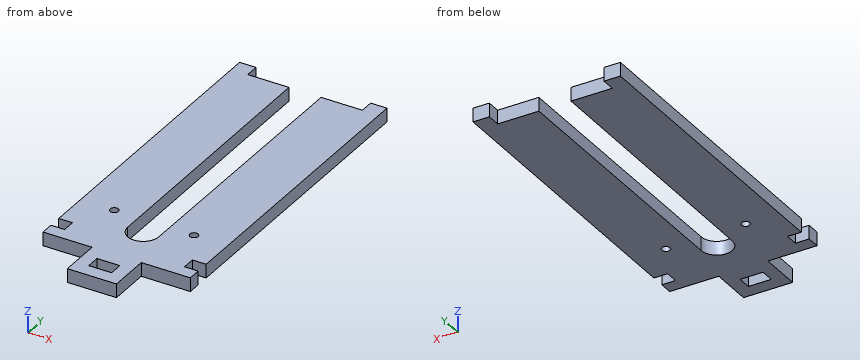
```python
from build123d import *

# Parameters (mm, degrees)
SKETCH1_W           = 57.15
SKETCH1_H           = 127
BOSS_EXTRUDE3_DEPTH = 5.334
CUT_EXTRUDE2_DEPTH  = 140.368483008
SKETCH8_W           = 19.05
SKETCH8_H           = 5.334
CUT_EXTRUDE6_DEPTH  = 5.334
SKETCH8_5_W         = 19.05
SKETCH8_5_H         = 5.334
CUT_EXTRUDE7_DEPTH  = 5.334
SKETCH16_W          = 22.352
SKETCH16_H          = 5.334
BOSS_EXTRUDE4_DEPTH = 5.334
SKETCH32_W          = 16.002
SKETCH32_H          = 5.334
CUT_EXTRUDE13_DEPTH = 5.334
SKETCH35_R          = 1.6
CUT_EXTRUDE15_DEPTH = 145.245837417
SKETCH36_W          = 19.05
SKETCH36_H          = 5.334
BOSS_EXTRUDE5_DEPTH = 10.668
SKETCH37_W          = 8.89
SKETCH37_H          = 5.334
CUT_EXTRUDE16_DEPTH = 145.245837417
SKETCH38_W          = 5.334
SKETCH38_H          = 5.08
CUT_EXTRUDE17_DEPTH = 145.245837417


with BuildPart() as part:
    # Sketch1 → Boss-Extrude3 (new body)
    with BuildSketch(Plane.XY):
        with Locations((28.575, 63.5)):
            Rectangle(SKETCH1_W, SKETCH1_H)
    extrude(amount=BOSS_EXTRUDE3_DEPTH)

    # Sketch3 → Cut-Extrude2 (cut, through all)
    with BuildSketch(Plane.XY.offset(5.334)):
        with BuildLine():
            Line((34.798, 127), (22.352, 127))
            Line((22.352, 127), (22.548184887, 22.479))
            ThreePointArc((22.548184887, 22.479), (28.575, 16.452184887), (34.601815113, 22.479))
            Line((34.601815113, 22.479), (34.798, 127))
        make_face()
    extrude(amount=-CUT_EXTRUDE2_DEPTH, mode=Mode.SUBTRACT)

    # Sketch8 → Cut-Extrude6 (cut)
    with BuildSketch(Plane.XZ):
        with Locations((47.625, 2.667)):
            Rectangle(SKETCH8_W, SKETCH8_H)
    extrude(amount=-CUT_EXTRUDE6_DEPTH, mode=Mode.SUBTRACT)

    # Sketch8<5> → Cut-Extrude7 (cut)
    with BuildSketch(Plane.XZ):
        with Locations((47.625, 2.667)):
            Rectangle(SKETCH8_5_W, SKETCH8_5_H)
        with Locations((9.525, 2.667)):
            Rectangle(SKETCH8_5_W, SKETCH8_5_H)
    extrude(amount=-CUT_EXTRUDE7_DEPTH, mode=Mode.SUBTRACT)

    # Sketch16 → Boss-Extrude4 (add)
    with BuildSketch(Plane(origin=(0, 127, 0), x_dir=(1, 0, 0), z_dir=(0, 1, 0))):
        with Locations((45.974, -2.667)):
            Rectangle(SKETCH16_W, SKETCH16_H)
        with Locations((11.176, -2.667)):
            Rectangle(SKETCH16_W, SKETCH16_H)
    extrude(amount=BOSS_EXTRUDE4_DEPTH)

    # Sketch32 → Cut-Extrude13 (cut)
    with BuildSketch(Plane(origin=(0, 132.334, 0), x_dir=(1, 0, 0), z_dir=(0, 1, 0))):
        with Locations((14.351, -2.667)):
            Rectangle(SKETCH32_W, SKETCH32_H)
        with Locations((42.799, -2.667)):
            Rectangle(SKETCH32_W, SKETCH32_H)
    extrude(amount=-CUT_EXTRUDE13_DEPTH, mode=Mode.SUBTRACT)

    # Sketch35 → Cut-Extrude15 (cut, through all)
    with BuildSketch(Plane.XY.offset(5.334)):
        with Locations((13.107594454, 29.550730033)):
            Circle(SKETCH35_R)
        with Locations((44.107261808, 29.40711974)):
            Circle(SKETCH35_R)
    extrude(amount=-CUT_EXTRUDE15_DEPTH, mode=Mode.SUBTRACT)

    # Sketch36 → Boss-Extrude5 (add)
    with BuildSketch(Plane.XZ):
        with Locations((28.575, 2.667)):
            Rectangle(SKETCH36_W, SKETCH36_H)
    extrude(amount=BOSS_EXTRUDE5_DEPTH)

    # Sketch37 → Cut-Extrude16 (cut, through all)
    with BuildSketch(Plane(origin=(0, 0, 0), x_dir=(-1, 0, 0), z_dir=(0, 0, -1))):
        with Locations((-28.575, -2.667)):
            Rectangle(SKETCH37_W, SKETCH37_H)
    extrude(amount=-CUT_EXTRUDE16_DEPTH, mode=Mode.SUBTRACT)

    # Sketch38 → Cut-Extrude17 (cut, through all)
    with BuildSketch(Plane(origin=(0, 0, 0), x_dir=(-1, 0, 0), z_dir=(0, 0, -1))):
        with Locations((-54.483, 12.954)):
            Rectangle(SKETCH38_W, SKETCH38_H)
        with Locations((-2.667, 12.954)):
            Rectangle(SKETCH38_W, SKETCH38_H)
    extrude(amount=-CUT_EXTRUDE17_DEPTH, mode=Mode.SUBTRACT)


solid = part.part
```
The listing builds one solid part. Answer for the finished solid, in the listing's coordinates (mm). Give positions to 0.01 mm unless a question says otherwise; leave off trailing zeros. Order: outer loops, then holes, each group sorted by start corner. A loop starts at its lowest first (then second) coordinate and runs counter-clockwise, first axis right, second up. Notation, with made-up numbers: (70, 50) - (99, 50) arc R23 ccw to (99, 88) - close; hole circle Ø5 at (79.5, 49.5). An arc over 180 degrees is marked (long way). Answer in a Markdown table with one row per item. Add a question column.
Q1. Given P1, Ø1.5, axis at y = 78.5, z = 2.5, coming from the -X side; P2, Ø1.6, axis at y = -1.5, z = 3.5, coming from the -X side; P3, Ø1.5, axis at y = 13.5, z = 2, coming from the +X side; P4, Ø2.5, axis at y = 13.5, z = 3, coming from the -X side, each flat-ended and moving along its own axis, determine where each tip first touches the part or whether it passes through.
Q2. Find the intervals of material crossed by line 1 along Y through (x, z) = (13, 4.35); line 2 along X through (y, z) = (113, 3); line 3 along Y through (x, z) = (5, 4.35), in increasing order. Write a range as [from, to].
Q3. The part is cut by section D-D (x = 47). Determine the outline of the cut face in (y, z).
Q4. The part is cut by section C-C (y = 72). Determine the outline of the cut face in (x, z), then the cut area to 3 significant figures.
Q5. The part is cut by section B-B (z = 3). Give the number of separate pieces and of enclosed holes in the cut face, then the cut area to 3 significant figures.
Q6. The part is cut by section A-A (y = 42). Determine the outline of the cut face in (x, z).
Determined:
| question | item | result |
|---|---|---|
| 1 | P1 | stops at x = 0 |
| 1 | P2 | stops at x = 19.05 |
| 1 | P3 | stops at x = 51.82 |
| 1 | P4 | stops at x = 5.33 |
| 2 | line 1 | y = [5.33, 27.95], [31.15, 127] |
| 2 | line 2 | x = [0, 22.38], [34.77, 57.15] |
| 2 | line 3 | y = [5.33, 10.41], [15.49, 132.33] |
| 3 | outline | (5.33, 0) - (127, 0) - (127, 5.33) - (5.33, 5.33) - close |
| 4 | outline | (0, 0) - (22.46, 0) - (22.46, 5.33) - (0, 5.33) - close; (34.69, 0) - (57.15, 0) - (57.15, 5.33) - (34.69, 5.33) - close |
| 4 | area | 240 mm² |
| 5 | separate pieces | 1 |
| 5 | enclosed holes | 3 |
| 5 | area | 5,870 mm² |
| 6 | outline | (0, 0) - (22.51, 0) - (22.51, 5.33) - (0, 5.33) - close; (34.64, 0) - (57.15, 0) - (57.15, 5.33) - (34.64, 5.33) - close |
